Check sheet for the modelled part. Datum: model origin and axes. Units: mm. A direction names the side the tool comes from. Round coordinates to 2 decimals unless told otherwise and drop trailing zeros. Order: outer loops, then holes, each group sorted by start corner. A loop starts at its lowest first (then second) coordinate and runs counter-clockwise, first axis right, second up.
(1) Depth check by flat-ended pin: pin 1 (1.5 mm diameter, centred on x = -53.5, y = 9.5, fed in from +Z); pin 2 (10 mm diameter, centred on x = -54.5, z = -69, fed in from -Y); pin 3 (2 mm diameter, centred on y = 29, z = -45, fed in from -X). Enter the tip coordinate at first touch or a pass-through.
(2) Sectioned sample at A-A, the plane x = -50.8. Enter the section's corners in (y, z).
(3) Sectioned sample at D-D, the plane z = -31. Enter the section's corners in (x, y).
(4) Sectioned sample at C-C, the plane y = 9.5. Enter the section's corners in (x, z), and give its area (3 significant figures).
(5) Thickness scan on probe 1 along Z at (x, y) = (-50.8, 3.65); probe 2 along Z at (x, y) = (-50.8, 24); probe 3 along Y at (x, z) = (-45.5, -70). Record the ranges inside material, lowest first.
(6) Mould release check, pull along Z, two halves, no side actions. Record for faces 4 (the cylindrical face through (-51.75, 3.8, -42.94)), 5 (the flat face through (-49, 14.922, -26)), 6 (the flat face through (-49, 9, -33.592)): released by +Z, released by -Z, zero draft, split by the parting line, or undercut.
(7) Sectioned sample at B-B, the plane z = -50.8. Enter the section's corners in (x, y), and give its area (3 significant figures).
(8) Tool access check on faces 1 (the cylindrical face through (-39.376, 12.614, -50.415)), 2 (the flat face through (-49, 2.54, -45)), 3 (the flat face through (-49, 9, -63.5)). Record the directions out of +Z, -Z, +X, -X, +Y, -Y that give a thin tool (end or side, any length) a straight path to the whole face; none if there is none.
Autodesk Inventor part; units mm, degrees
ref_plane "YZ Plane" through (0, 0, 0) normal (1, 0, 0) x (0, 1, 0)
ref_plane "XZ Plane" through (0, 0, 0) normal (0, 1, 0) x (-1, 0, 0)
ref_plane "XY Plane" through (0, 0, 0) normal (0, 0, 1) x (1, 0, 0)
sketch "Sketch1" plane through (0, 0, 0) normal (0, 1, 0) x (-1, 0, 0)
  line L0 (0, 0) -> (101.6, 0)
  line L1 (101.6, 0) -> (101.6, -101.6)
  line L2 (101.6, -101.6) -> (0, -101.6)
  line L3 (0, -101.6) -> (0, 0)
  circle A0 centre (50.8, -50.8) radius 5.461
  dimension "d0" = 101.6
  dimension "d1" = 101.6
  dimension "d2" = 10.922
extrude "Extrusion1" add sketch "Sketch1" along normal blind 4.7625
sketch "Sketch2" plane through (0, 4.7625, 0) normal (0, 1, 0) x (1, 0, 0)
  line L0 (-101.6, 0) -> (0, 0)
  line L1 (-76.2, 0) -> (0, 0)
  line L2 (0, 0) -> (0, 33.5923)
  line L3 (0, 33.5923) -> (-76.2, 33.5923)
  line L4 (-76.2, 33.5923) -> (-76.2, 0)
  line L5 (-101.6, 101.6) -> (-101.6, 0)
  line L6 (0, 0) -> (0, 101.6)
  line L7 (0, 101.6) -> (-101.6, 101.6)
  line L8 (-101.6, 76.2) -> (0, 76.2)
  line L9 (0, 76.2) -> (0, 101.6)
  line L10 (0, 101.6) -> (-101.6, 101.6)
  line L11 (-101.6, 101.6) -> (-101.6, 76.2)
  circle A0 centre (-50.8, 50.8) radius 5.461
  line L12 (0, 76.2) -> (-38.1, 76.2)
  line L13 (-38.1, 76.2) -> (-38.1, 33.5923)
  line L14 (-38.1, 33.5923) -> (0, 33.5923)
  line L15 (0, 33.5923) -> (0, 76.2)
  point P0 (0, 76.2)
  dimension "d5" = 25.4
  dimension "d6" = 0
  dimension "d9" = 25.4
extrude "Extrusion2" cut sketch "Sketch2" against normal through all contours L4 L3 L2 L0 | L5 L7 L6 L8 | L8 L6 L3 L13
sketch "Sketch3" plane through (0, 4.7625, 0) normal (0, 1, 0) x (1, 0, 0)
  line L0 (-93.6015, 4.7625) -> (-89.5375, 4.7625)
  line L1 (-89.5375, 4.7625) -> (-89.5375, 71.4375)
  line L2 (-89.5375, 71.4375) -> (-93.6015, 71.4375)
  line L3 (-93.6015, 71.4375) -> (-93.6015, 4.7625)
  line L4 (-101.6, 0) -> (-76.2, 0)
  line L5 (-101.6, 76.2) -> (-101.6, 0)
  line L6 (-38.1, 76.2) -> (-101.6, 76.2)
  line L7 (-83.6041, 71.4375) -> (-83.6041, 4.7625)
  line L8 (-79.5401, 71.4375) -> (-83.6041, 71.4375)
  line L9 (-79.5401, 4.7625) -> (-79.5401, 71.4375)
  line L10 (-83.6041, 4.7625) -> (-79.5401, 4.7625)
  line L11 (-73.6067, 71.4375) -> (-73.6067, 4.7625)
  line L12 (-69.5427, 71.4375) -> (-73.6067, 71.4375)
  line L13 (-69.5427, 4.7625) -> (-69.5427, 71.4375)
  line L14 (-73.6067, 4.7625) -> (-69.5427, 4.7625)
  line L15 (-63.6092, 71.4375) -> (-63.6092, 4.7625)
  line L16 (-59.5452, 71.4375) -> (-63.6092, 71.4375)
  line L17 (-59.5452, 4.7625) -> (-59.5452, 71.4375)
  line L18 (-63.6092, 4.7625) -> (-59.5452, 4.7625)
  point P0 (0, 0)
  dimension "d10" = 4.064
  dimension "d11" = 4.7625
  dimension "d12" = 7.9985
  dimension "d14" = 4.7625
  dimension "d17" = 9.9974
extrude "Extrusion3" cut sketch "Sketch3" against normal through all
sketch "Sketch4" plane through (0, 4.7625, 0) normal (0, 1, 0) x (1, 0, 0)
  circle A0 centre (-50.8, 42.9006) radius 0.9525
  circle A1 centre (-50.8, 50.8) radius 5.461
  point P0 (0, 0)
  dimension "d24" = 1.905
  dimension "d25" = 0
  dimension "d26" = 7.8994
extrude "Extrusion4" cut sketch "Sketch4" against normal through all contours A0
sketch "Sketch5" plane through (0, 4.7625, 0) normal (0, 1, 0) x (1, 0, 0)
  line L0 (-101.6, 0) -> (-76.2, 0)
  line L1 (-38.1, 76.2) -> (-101.6, 76.2)
  line L2 (-101.6, 0) -> (-59.2938, 0)
  line L3 (-59.2938, 0) -> (-59.2938, 76.2)
  line L4 (-59.2938, 76.2) -> (-101.6, 76.2)
  line L5 (-101.6, 76.2) -> (-101.6, 0)
  point P0 (0, 0)
extrude "Extrusion5" cut sketch "Sketch5" against normal through all
sketch "Sketch6" plane through (0, 4.7625, 0) normal (0, 1, 0) x (1, 0, 0)
  circle A0 centre (-50.8, 50.8) radius 5.461
  line L0 (-59.2938, 76.2) -> (-59.2938, 33.5923)
  line L1 (-59.2938, 33.5923) -> (-38.1, 33.5923)
  line L2 (-38.1, 33.5923) -> (-38.1, 76.2)
  line L3 (-38.1, 76.2) -> (-59.2938, 76.2)
  circle A1 centre (-50.8, 42.9006) radius 0.9525
  point P0 (0, 0)
extrude "Extrusion6" add sketch "Sketch6" along normal blind 15.24
sketch "Sketch7" plane through (0, 20.0025, 0) normal (0, 1, 0) x (1, 0, 0)
  circle A0 centre (-50.8, 50.8) radius 5.461
  circle A1 centre (-50.8, 50.8) radius 11.43
  point P0 (0, 0)
  dimension "d33" = 22.86
extrude "Extrusion7" cut sketch "Sketch7" against normal blind 14.986
sketch "Sketch10" plane through (0, 0, 0) normal (0, -1, 0) x (1, 0, 0)
  line L0 (-59.2938, -76.2) -> (-38.1, -76.2)
  line L1 (-38.1, -76.2) -> (-38.1, -33.5923)
  line L2 (-59.2938, -76.2) -> (-38.1, -76.2)
  line L3 (-38.1, -76.2) -> (-38.1, -63.5)
  line L4 (-38.1, -63.5) -> (-59.2938, -63.5)
  line L5 (-59.2938, -63.5) -> (-59.2938, -76.2)
  point P0 (0, 0)
  dimension "d36" = 12.7
extrude "Extrusion8" cut sketch "Sketch10" against normal blind 14.986
sketch "Sketch11" plane through (-59.2938, 0, -33.5923) normal (0, 0, 1) x (1, 0, 0)
  line L0 (21.1938, 20.0025) -> (0, 20.0025)
  line L1 (21.1938, 20.0025) -> (21.1938, 14.986)
  line L2 (0, 20.0025) -> (21.1938, 20.0025)
  line L3 (21.1938, 20.0025) -> (21.1938, 14.9225)
  line L4 (21.1938, 14.9225) -> (0, 14.9225)
  line L5 (0, 14.9225) -> (0, 20.0025)
  point P0 (59.2938, 0)
  point P1 (21.1938, 14.986)
  dimension "d39" = 5.08
extrude "Extrusion9" add sketch "Sketch11" along normal blind 14.986
sketch "Sketch12" plane through (0, 0, 0) normal (0, -1, 0) x (1, 0, 0)
  line L0 (-59.2938, -63.5) -> (-38.1, -63.5)
  line L1 (-38.1, -63.5) -> (-38.1, -33.5923)
  line L2 (-38.1, -33.5923) -> (-59.2938, -33.5923)
  line L3 (-59.2938, -33.5923) -> (-59.2938, -63.5)
  circle A0 centre (-50.8, -42.9006) radius 0.9525
  circle A1 centre (-50.8, -50.8) radius 5.461
  point P0 (0, 0)
extrude "Extrusion10" cut sketch "Sketch12" against normal blind 2.54
sketch "Sketch13" plane through (0, 20.0025, 0) normal (0, 1, 0) x (1, 0, 0)
  arc A0 (-59.2938, 43.1515) -> (-59.2938, 58.4485) centre (-50.8, 50.8) ccw
  line L0 (-59.2938, 43.1515) -> (-59.2938, 18.6063)
  line L1 (-38.1, 18.6063) -> (-59.2938, 18.6063)
  line L2 (-38.1, 76.2) -> (-38.1, 18.6063)
  line L3 (-38.1, 76.2) -> (-59.2938, 76.2)
  line L4 (-59.2938, 76.2) -> (-59.2938, 58.4485)
  point P0 (0, 0)
extrude "Extrusion11" add sketch "Sketch13" along normal blind 13.716
properties part number "rotary encoder mount"
Derived:
1. pin 1: stops at z = -33.59
1. pin 2: stops at y = 14.99
1. pin 3: stops at x = -41.61
2. outline: (2.54, -63.5) - (14.99, -63.5) - (14.99, -76.2) - (33.72, -76.2) - (33.72, -62.23) - (5.02, -62.23) - (5.02, -56.26) - (2.54, -56.26) - close; (2.54, -45.34) - (5.02, -45.34) - (5.02, -43.85) - (2.54, -43.85) - close; (2.54, -41.95) - (5.02, -41.95) - (5.02, -39.37) - (33.72, -39.37) - (33.72, -18.61) - (14.92, -18.61) - (14.92, -33.59) - (2.54, -33.59) - close
3. outline: (-59.29, 14.92) - (-38.1, 14.92) - (-38.1, 33.72) - (-59.29, 33.72) - close
4. outline: (-59.29, -63.5) - (-38.1, -63.5) - (-38.1, -33.59) - (-59.29, -33.59) - (-59.29, -43.15) arc R11.43 cw (long way) to (-59.29, -58.45) - close
4. area: 254 mm2
5. probe 1: z = -63.5 to -56.26, -45.34 to -43.85, -41.95 to -33.59
5. probe 2: z = -76.2 to -62.23, -39.37 to -18.61
5. probe 3: y = 14.99 to 33.72
6. face 4: undercut
6. face 5: zero draft
6. face 6: released by +Z
7. outline: (-59.29, 2.54) - (-56.26, 2.54) - (-56.26, 5.02) - (-59.29, 5.02) - close; (-45.34, 2.54) - (-38.1, 2.54) - (-38.1, 33.72) - (-39.37, 33.72) - (-39.37, 5.02) - (-45.34, 5.02) - close
7. area: 61.9 mm2
8. face 1: +Y
8. face 2: +Z, -Z, +X, -X, -Y
8. face 3: -Z, +X, -X, -Y
